Source: CAD feature listing. Evaluate the final solid. Frame: model axes, mm. Face numbers are marked on the shaded views. Coordinates: 2 decimals unless noted, no trailing zeros. Write each loop counter-clockwise with the first axis right and the second up, starting at its lowest first coordinate (ties: lowest second). Pieces come first, ordered by that corner, then holes. Notation, with made-up numbers: (53, 7.25) - (86, 7.25) arc R14 ccw to (86, 28.25) - close; hole circle Ø9 at (75.25, 65.25). An arc over 180 degrees is marked (long way). One line per item, written item: value.
from build123d import *


with BuildPart() as part:
    # Sketch1 → Revolve1 (revolve)
    with BuildSketch(Plane(origin=(0, 0, 0), x_dir=(1, 0, 0), z_dir=(0, 1, 0))):
        with BuildLine():
            Line((1.571907147, 25), (1.571907147, 26))
            Line((1.571907147, 26), (-0.428092853, 26))
            Line((-0.428092853, 26), (-0.428092853, 25))
            Line((-0.428092853, 25), (-3.428092853, 25))
            Line((-3.428092853, 25), (-3.428092853, 23))
            Line((-3.428092853, 23), (0.338990058, 21.425225269))
            ThreePointArc((0.338990058, 21.425225269), (2.644708452, 18.573477692), (3.468758659, 15))
            Line((3.468758659, 15), (5.468758659, 15))
            ThreePointArc((5.468758659, 15), (4.4427399, 19.449310388), (1.571907147, 23))
            Line((1.571907147, 23), (1.571907147, 25))
        make_face()
    revolve(axis=Axis((-17.365592853, 0, 0), (1, 0, 0)))


solid = part.part
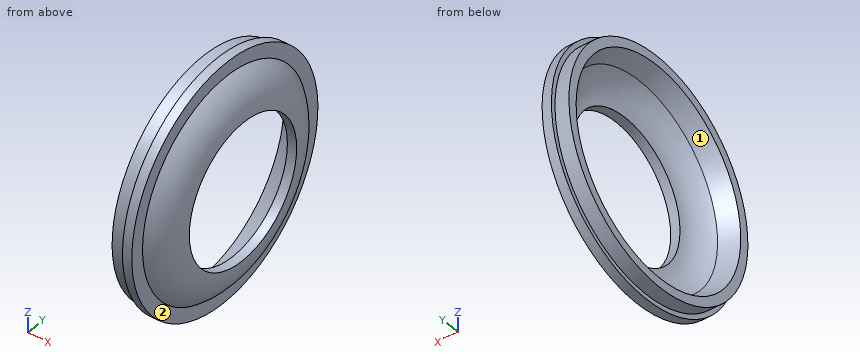
1) Contact query for flat-ended pins moving along their axis: P1, Ø2, axis at x = -2, z = -3, coming from the +Y side; P2, Ø4, axis at x = -0.5, y = 19, coming from the +Z side; P3, Ø15.5, axis at y = 4.5, z = 4.5, coming from the +X side. Output: stop coordinate, or through.
Values found:
P1: y = 24.92
P2: z = 19.67
P3: through
2) Material intervals for line 1 (Y direction, x = 1.25, z = -6); line 2 (Y direction, x = 4.55, z = 0); line 3 (Z direction, x = 2, y = -16), sorted ascending.
Values found:
line 1: -25.3 to -19.7, 19.7 to 25.3
line 2: -19.22 to -15, 15 to 19.22
line 3: -16.03 to -11.44, 11.44 to 16.03
3) Section query C-C on x = -1.5. Output: boundary loops of the cut face in (y, z), then the cut area to 3 significant figures.
Values found:
outline: circle Ø50 at (0, 0); hole circle Ø44.39 at (0, 0)
area: 416 mm2
4) Draft query along Z for the marked faces 1 and 2. Return one class per face: released by +Z, released by -Z, zero draft, split by the parting line, or undercut.
Values found:
face 1: undercut
face 2: zero draft
5) Section query A-A on z = 0. Output: boundary loops of the cut face in (x, y), then the cut area to 3 significant figures.
Values found:
outline: (-3.43, -25) - (-0.43, -25) - (-0.43, -26) - (1.57, -26) - (1.57, -23) arc R10.16 ccw to (5.47, -15) - (3.47, -15) arc R8.16 cw to (0.34, -21.43) - (-3.43, -23) - close; (-3.43, 23) - (0.34, 21.43) arc R8.16 cw to (3.47, 15) - (5.47, 15) arc R10.16 ccw to (1.57, 23) - (1.57, 26) - (-0.43, 26) - (-0.43, 25) - (-3.43, 25) - close
area: 65.1 mm2
